Answer from the drawing. Dimensions are ordinates in mm from the lowest x, y and z of the part. A direction names the side the tool comes from. Round coordinates to 2 decimals unless told otherwise and drop trailing zeros. Loops run counter-clockwise (first coordinate to the right, second up) from the corner with the lowest first, then second, coordinate; pieces in that order, holes last. Notation, with made-up numbers: (-1.5, 51) - (40.5, 51) arc R26 cw to (40.5, 80) - close; hole circle Ø2 at (82.25, 48.25). An arc over 180 degrees is marked (long way). Answer as CSV lines item,"result".
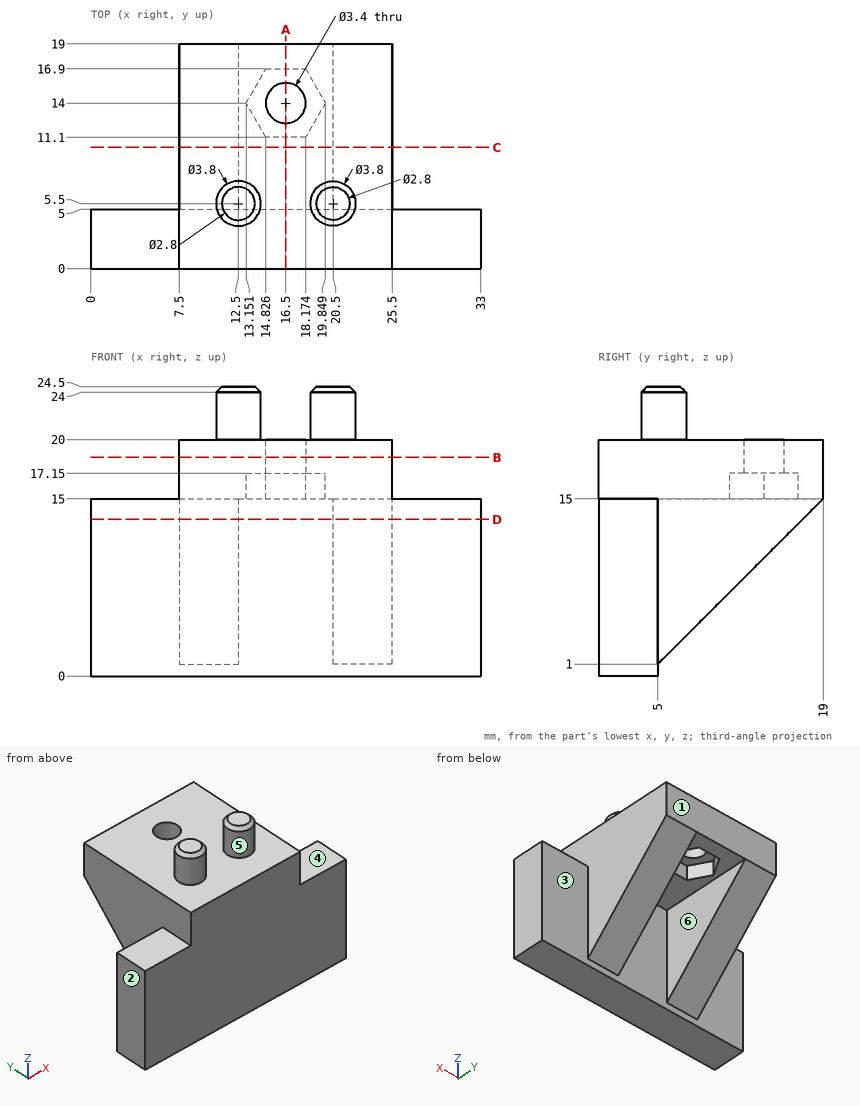
1) Each of these flat-tipped pins is pushed along its axis until it touches: P1, Ø7.5, axis at x = 14.5, z = 10.5, coming from the +Y side; P2, Ø4, axis at y = 13.5, z = 9, coming from the -X side; P3, Ø4.5, axis at x = 16.5, y = 14, coming from the -Z side. Where does it stop, or does it pass through?
Entries:
P1,"stops at y = 17.67"
P2,"stops at x = 7.5"
P3,"stops at z = 17.15"
2) A cutting plane is placed at C-C, the plane y = 10.25. Determine the outline of the cut face in (x, z).
Entries:
outline,"(7.5, 6.25) - (12.5, 6.25) - (12.5, 15) - (20.5, 15) - (20.5, 6.25) - (25.5, 6.25) - (25.5, 20) - (7.5, 20) - close"
3) A cutting plane is placed at B-B, the plane z = 18.5. Determine the outline of the cut face in (x, y).
Entries:
outline,"(7.5, 0) - (25.5, 0) - (25.5, 19) - (7.5, 19) - close; hole circle Ø3.4 at (16.5, 14)"
4) The mould has two halves that part along X. Classify the marked faces 1, 2 and 3: pulls with the +X half, pulls with the -X half, needs draft (parallel to the pull), parting line crosses it, or undercut.
Entries:
face 1,"needs draft"
face 2,"pulls with the -X half"
face 3,"undercut"
5) A cutting plane is placed at A-A, the plane x = 16.5. Determine the outline of the cut face in (y, z), plus the area to 3 significant figures.
Entries:
outline,"(0, 0) - (5, 0) - (5, 15) - (11.1, 15) - (11.1, 17.15) - (12.3, 17.15) - (12.3, 20) - (0, 20) - close; (15.7, 17.15) - (16.9, 17.15) - (16.9, 15) - (19, 15) - (19, 20) - (15.7, 20) - close"
area,"148 mm^2"
6) A tool of negligible diameter and unlimited length cuts with its end or side. For the marked faces 4, 5 and 6, from which of +Z, -Z, +X, -X, +Y, -Y can it reach the whole face along a straight path? Write none if from no direction.
Entries:
face 4,"+Z, +X, +Y, -Y"
face 5,"+Z"
face 6,"-Z, +Y"
7) A cutting plane is placed at D-D, the plane z = 13.25. Determine the outline of the cut face in (x, y).
Entries:
outline,"(0, 0) - (33, 0) - (33, 5) - (25.5, 5) - (25.5, 17.25) - (20.5, 17.25) - (20.5, 5) - (12.5, 5) - (12.5, 17.25) - (7.5, 17.25) - (7.5, 5) - (0, 5) - close"
8) Find the intervals of material crossed by line 1 (X direction, y = 9.5, z = 11); line 2 (Y direction, x = 16.5, z = 18.9); line 3 (X direction, y = 14.75, z = 16.75) (1 decimal), in increasing order.
Entries:
line 1,"x = 7.5 to 12.5, 20.5 to 25.5"
line 2,"y = 0 to 12.3, 15.7 to 19"
line 3,"x = 7.5 to 13.6, 19.4 to 25.5"
